Autodesk Fusion 360 part; units mm, degrees
sketch "Sketch1" plane through (0, 0, 0) normal (0, 0, 1) x (1, 0, 0)
  line L0 (-51.0433, -16.8971) -> (557.9567, -16.8971)
  line L1 (557.9567, -16.8971) -> (557.9567, 287.1029)
  line L2 (557.9567, 287.1029) -> (-51.0433, 287.1029)
  line L3 (-51.0433, 287.1029) -> (-51.0433, -16.8971)
  line L4 (-41.0433, -6.8971) -> (547.9567, -6.8971)
  line L5 (547.9567, -6.8971) -> (547.9567, 277.1029)
  line L6 (547.9567, 277.1029) -> (-41.0433, 277.1029)
  line L7 (-41.0433, 277.1029) -> (-41.0433, -6.8971)
  line L8 (-61.0433, -26.8971) -> (567.9567, -26.8971)
  line L9 (567.9567, -26.8971) -> (567.9567, 297.1029)
  line L10 (567.9567, 297.1029) -> (-61.0433, 297.1029)
  line L11 (-61.0433, 297.1029) -> (-61.0433, -26.8971)
  circle A0 centre (-55.5433, -21.3971) radius 5
  circle A1 centre (-55.5433, 291.6029) radius 5
  circle A2 centre (562.4567, 291.6029) radius 5
  circle A3 centre (562.4567, -21.3971) radius 5
  dimension "d1" = 609
  dimension "d2" = 304
  dimension "d3" = 10
  dimension "d4" = 10
  dimension "d5" = 10
  dimension "d6" = 10
  dimension "d7" = 10
  dimension "d8" = 10
  dimension "d9" = 10
  dimension "d10" = 10
  dimension "d11" = 10
  dimension "d12" = 5.5
  dimension "d13" = 5.5
  dimension "d14" = 10
  dimension "d15" = 5.5
  dimension "d16" = 5.5
  dimension "d17" = 10
  dimension "d18" = 5.5
  dimension "d19" = 5.5
  dimension "d20" = 10
  dimension "d21" = 5.5
  dimension "d22" = 5.5
extrude "Extrude1" add sketch "Sketch1" along normal blind 5 contours L0 L1 L2 L3
extrude "Extrude2" add sketch "Sketch1" along normal blind 50 contours L8 L9 L10 L11
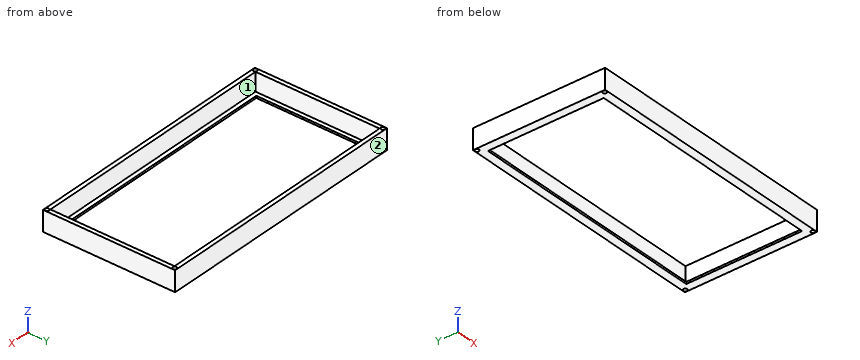
Could you check a few things on this model? Use its own coordinates, in mm. Face numbers are marked on the shaded views. A direction names the side the tool comes from. Give positions to 0.01 mm unless a question says otherwise; leave off trailing zeros. Order: outer loops, then holes, each group sorted by start corner. A loop starts at its lowest first (then second) coordinate and runs counter-clockwise, first axis right, second up.
1. Suppose I cut it at B-B (x = 319). List the corners of the cut face in (y, z) for me.
2. For the marked faces 1 and 2, which set-ups out of +Z, -Z, +X, -X, +Y, -Y let a thin tool reach every point of the face, with its end or its side?
3. Suppose I cut it at A-A (y = 29.5). List the corners of the cut face in (x, z) for me.
4. Will this pin go through, and if not, where does the flat tip stop? P1, Ø16, axis at x = 562.46, y = -21.4, coming from the +Z side.
5. I need wall thicknesses on L1, parallel to Y at x = 478, z = 48; L2, parallel to X at y = -4, z = 4.5; L3, parallel to X at y = 137, z = 25. Which ranges of each line are inside material? Lowest first, please.
6. Suppose I cut it at C-C (z = 40). List the corners of the cut face in (x, y) for me, plus the area to 3 significant figures.
Solved:
1. outline: (-26.9, 0) - (-6.9, 0) - (-6.9, 5) - (-16.9, 5) - (-16.9, 50) - (-26.9, 50) - close; (277.1, 0) - (297.1, 0) - (297.1, 50) - (287.1, 50) - (287.1, 5) - (277.1, 5) - close
2. face 1: +Z
2. face 2: +Z, -Z, +X, -X, +Y
3. outline: (-61.04, 0) - (-41.04, 0) - (-41.04, 5) - (-51.04, 5) - (-51.04, 50) - (-61.04, 50) - close; (547.96, 0) - (567.96, 0) - (567.96, 50) - (557.96, 50) - (557.96, 5) - (547.96, 5) - close
4. P1: stops at z = 50
5. L1: y = -26.9 to -16.9, 287.1 to 297.1
5. L2: x = -61.04 to -41.04, 547.96 to 567.96
5. L3: x = -61.04 to -51.04, 557.96 to 567.96
6. outline: (-61.04, -26.9) - (567.96, -26.9) - (567.96, 297.1) - (-61.04, 297.1) - close; hole circle Ø10 at (-55.54, -21.4); hole circle Ø10 at (-55.54, 291.6); hole (-51.04, -16.9) - (557.96, -16.9) - (557.96, 287.1) - (-51.04, 287.1) - close; hole circle Ø10 at (562.46, -21.4); hole circle Ø10 at (562.46, 291.6)
6. area: 18,300 mm2
